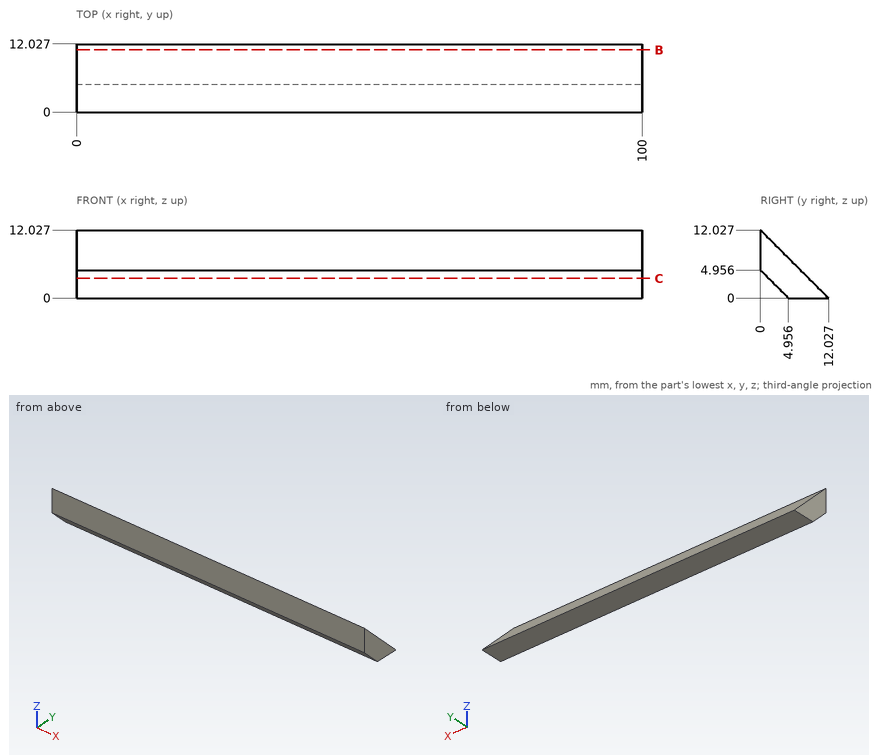
For this review, use the dimensioned drawing (mm, ordinates from the lowest corner) and the shaded views. Give positions to 0.01 mm unless a question says otherwise; leave off trailing zeros. Order: outer loops, then holes, each group sorted by start corner. A loop starts at its lowest first (then second) coordinate and runs counter-clockwise, first axis right, second up. Notation, with made-up numbers: (86.5, 22.25) - (121.5, 22.25) arc R10 cw to (121.5, 35.25) - close; hole circle Ø8 at (71.5, 86). An arc over 180 degrees is marked (long way). Use a Markdown table: item, result. Add a question column.
(1) Wall thickness on probe 1 along Z at (x, y) = (12, 7) (1 decimal); probe 2 along Z at (x, y) = (27.5, 3) (1 decimal); probe 3 along Y at (x, z) = (86.5, 10) (1 decimal): over which ranges is each line inside the solid? List them lowest first. Write a range as [from, to].
(2) Clearance check with flat-ended pins moving along their axes: P1, Ø2, axis at x = 28, z = 4.5, coming from the -Y side; P2, Ø1, axis at x = 57.5, y = 6, coming from the +Z side (1 decimal); P3, Ø6, axis at x = 67, y = 8, coming from the +Z side (1 decimal). State where each tip first meets the part, or that it passes through.
(3) Add section B-B on y = 11. Give the boundary of the cut face in (x, z).
(4) Add section C-C on z = 3.5. Give the boundary of the cut face in (x, y) (1 decimal).
Report:
| question | item | result |
|---|---|---|
| 1 | probe 1 | z = [0, 5] |
| 1 | probe 2 | z = [2, 9] |
| 1 | probe 3 | y = [0, 2] |
| 2 | P1 | stops at y = 0 |
| 2 | P2 | stops at z = 6.5 |
| 2 | P3 | stops at z = 7 |
| 3 | outline | (0, 0) - (100, 0) - (100, 1.03) - (0, 1.03) - close |
| 4 | outline | (0, 1.5) - (100, 1.5) - (100, 8.5) - (0, 8.5) - close |
